```python
from build123d import *

# Parameters (mm, degrees)
SKETCH025_R  = 1.7
PAD021_DEPTH = 100
BOX004_W     = 36
BOX004_H     = 7
BOX004_DEPTH = 2
BOX003_W     = 18
BOX003_H     = 45
BOX003_DEPTH = 2
BOX005_W     = 36
BOX005_H     = 7
BOX005_DEPTH = 2
BOX002_W     = 36
BOX002_H     = 20
BOX002_DEPTH = 2


with BuildPart() as pad021:
    # Sketch025 → Pad021 (new body)
    with BuildSketch(Plane.XY.offset(-50)):
        with Locations((0, -19)):
            Circle(SKETCH025_R)
        with Locations((-14.3, 16)):
            Circle(SKETCH025_R)
        with Locations((14.3, 16)):
            Circle(SKETCH025_R)
    extrude(amount=PAD021_DEPTH)


with BuildPart() as chassis003:
    # Box004 → Box004 (new body)
    with BuildSketch(Plane(origin=(-18, 13, -14.4), x_dir=(1, 0, 0), z_dir=(0, 0, 1))):
        with Locations((18, 3.5)):
            Rectangle(BOX004_W, BOX004_H)
    extrude(amount=BOX004_DEPTH)


with BuildPart() as chassis002:
    # Box003 → Box003 (new body)
    with BuildSketch(Plane(origin=(-9, -25, -14.4), x_dir=(1, 0, 0), z_dir=(0, 0, 1))):
        with Locations((9, 22.5)):
            Rectangle(BOX003_W, BOX003_H)
    extrude(amount=BOX003_DEPTH)


with BuildPart() as chassis004:
    # Box005 → Box005 (new body)
    with BuildSketch(Plane(origin=(-18, -25, -14.4), x_dir=(1, 0, 0), z_dir=(0, 0, 1))):
        with Locations((18, 3.5)):
            Rectangle(BOX005_W, BOX005_H)
    extrude(amount=BOX005_DEPTH)


with BuildPart() as cut005:
    # Box002 → Box002 (new body)
    with BuildSketch(Plane(origin=(-18, -12.5, -14.4), x_dir=(1, 0, 0), z_dir=(0, 0, 1))):
        with Locations((18, 10)):
            Rectangle(BOX002_W, BOX002_H)
    extrude(amount=BOX002_DEPTH)

    # Fusion002: union chassis003, chassis002, chassis004
    add(chassis003.part)
    add(chassis002.part)
    add(chassis004.part)

    # Cut005: cut Pad021
    add(pad021.part, mode=Mode.SUBTRACT)


solid = cut005.part
```
Geometry check sheet. Reference: the model listing, model coordinates, mm. A direction names the side the tool comes from. Round coordinates to 2 decimals unless told otherwise and drop trailing zeros. Loops run counter-clockwise (first coordinate to the right, second up) from the corner with the lowest first, then second, coordinate; pieces in that order, holes last. Notation, with made-up numbers: (-35.5, 33.25) - (-24.5, 33.25) arc R29 cw to (-24.5, 60.25) - close; hole circle Ø8 at (43.5, 34). An arc over 180 degrees is marked (long way). Write each question's results on one line, items separated by ' | '. Start each with the question number.
Q1. Cross-section at D-D on y = 15. Enter the section's corners in (x, z), and give its area (3 significant figures).
Q2. Cross-section at C-C on z = -13. Enter the section's corners in (x, y).
Q3. Gauge pin test, flat end, axial feed: P1, Ø1, axis at y = 10.5, z = -13.5, coming from the -X side. Record the tip position at first contact, or that the pin passes through.
Q4. Release check for a two-part mould opening along Y. For faces 1 (the flat face through (18, -22, -13)), 2 (the flat face through (0, 20, -13)), 3 (the flat face through (-14, 7.5, -13)) record: +Y half, -Y half, draft (parallel to the pull), parting line (faces both ways), or undercut.
Q5. Cross-section at B-B on x = 14.3. Enter the section's corners in (y, z), and give its area (3 significant figures).
Q6. Access from +Z, -Z, +X, -X, +Y, -Y to the whole of each face (thin tool, end or side, straight path). Record for faces 4 (the flat face through (-14, 13, -13)), 5 (the flat face through (0, -25, -13)), 6 (the flat face through (13, -18, -13)).
Q7. Cross-section at A-A on y = -19. Enter the section's corners in (x, z).
Q8. Thickness scan on line 1 (X direction, y = 16, z = -13.4); line 2 (Y direction, x = -14.3, z = -13.75); line 3 (X direction, y = 17, z = -13). Record the ranges inside material, lowest first. Write a range as [from, to].
Answers below:
1) outline: (-18, -14.4) - (-15.67, -14.4) - (-15.67, -12.4) - (-18, -12.4) - close; (-12.93, -14.4) - (12.93, -14.4) - (12.93, -12.4) - (-12.93, -12.4) - close; (15.67, -14.4) - (18, -14.4) - (18, -12.4) - (15.67, -12.4) - close | area: 61.0 mm²
2) outline: (-18, -25) - (18, -25) - (18, -18) - (9, -18) - (9, -12.5) - (18, -12.5) - (18, 7.5) - (9, 7.5) - (9, 13) - (18, 13) - (18, 20) - (-18, 20) - (-18, 13) - (-9, 13) - (-9, 7.5) - (-18, 7.5) - (-18, -12.5) - (-9, -12.5) - (-9, -18) - (-18, -18) - close; hole circle Ø3.4 at (-14.3, 16); hole circle Ø3.4 at (0, -19); hole circle Ø3.4 at (14.3, 16)
3) P1: stops at x = -9
4) face 1: draft | face 2: +Y half | face 3: undercut
5) outline: (-25, -14.4) - (-18, -14.4) - (-18, -12.4) - (-25, -12.4) - close; (-12.5, -14.4) - (7.5, -14.4) - (7.5, -12.4) - (-12.5, -12.4) - close; (13, -14.4) - (14.3, -14.4) - (14.3, -12.4) - (13, -12.4) - close; (17.7, -14.4) - (20, -14.4) - (20, -12.4) - (17.7, -12.4) - close | area: 61.2 mm²
6) face 4: +Z, -Z, -X | face 5: +Z, -Z, +X, -X, -Y | face 6: +Z, -Z, +X
7) outline: (-18, -14.4) - (-1.7, -14.4) - (-1.7, -12.4) - (-18, -12.4) - close; (1.7, -14.4) - (18, -14.4) - (18, -12.4) - (1.7, -12.4) - close
8) line 1: x = [-18, -16], [-12.6, 12.6], [16, 18] | line 2: y = [-25, -18], [-12.5, 7.5], [13, 14.3], [17.7, 20] | line 3: x = [-18, -15.67], [-12.93, 12.93], [15.67, 18]
